from build123d import *

# Parameters (mm, degrees)
SKETCH1_W           = 5
SKETCH1_H           = 25
BOSS_EXTRUDE1_DEPTH = 258.5
SKETCH2_R           = 3
SKETCH2_R_2         = 1.5
CUT_EXTRUDE1_DEPTH  = 259.850342862


with BuildPart() as part:
    # Sketch1 → Boss-Extrude1 (new body)
    with BuildSketch(Plane.XY):
        Rectangle(SKETCH1_W, SKETCH1_H)
    extrude(amount=BOSS_EXTRUDE1_DEPTH)

    # Sketch2 → Cut-Extrude1 (cut, through all)
    with BuildSketch(Plane(origin=(2.5, 0, 0), x_dir=(0, 0, -1), z_dir=(1, 0, 0))):
        with Locations((-12.5, 0)):
            Circle(SKETCH2_R)
        with Locations((-246, 0)):
            Circle(SKETCH2_R_2)
        with Locations((-228, 0)):
            Circle(SKETCH2_R_2)
        with Locations((-48.5, 0)):
            Circle(SKETCH2_R_2)
        with Locations((-31.5, 0)):
            Circle(SKETCH2_R_2)
        with BuildLine():
            Line((-12.5, 12.5), (5.5, 12.5))
            Line((5.5, 12.5), (5.5, -12.5))
            Line((5.5, -12.5), (-12.5, -12.5))
            ThreePointArc((-12.5, -12.5), (0, 0), (-12.5, 12.5))
        make_face()
        Polygon((-257.716878365, 0), (-250.5, 12.5), (-258.5, 12.5), (-258.5, -12.5), (-250.5, -12.5), align=None)
    extrude(amount=-CUT_EXTRUDE1_DEPTH, mode=Mode.SUBTRACT)


solid = part.part
Design review of the part built by this model. Coordinates are the model's own, in mm. Coordinates: 2 decimals unless noted, no trailing zeros. Loops run counter-clockwise (first coordinate to the right, second up) from the corner with the lowest first, then second, coordinate; pieces in that order, holes last. Notation, with made-up numbers: (1.25, 88.5) - (11.25, 88.5) arc R12 ccw to (11.25, 95.5) - close; hole circle Ø2 at (63.5, 35). An arc over 180 degrees is marked (long way). Use CSV: the item, a comma, the result in double quotes. Start each with the question number.
1. Clearance check with flat-ended pins moving along their axes: pin 1 (1 mm diameter, centred on x = -0.5, y = -2.5, fed in from -Z); pin 2 (5.5 mm diameter, centred on y = 0, z = 12.5, fed in from +X); pin 3 (1 mm diameter, centred on x = 0, y = 8.5, fed in from +Z); pin 4 (1.5 mm diameter, centred on x = 2, y = -1.5, fed in from -Z). State where each tip first meets the part, or that it passes through.
2. Mouldability with a two-part tool opening along Y and no side actions: class faces 1 (the cylindrical face through (0, -1.8, 14.9)), 2 (the flat face through (0.035, -6.337, 254.058)), 3 (the flat face through (-2.5, 0, 127)) as released by +Y, released by -Y, zero draft, split by the parting line, or undercut.
3. Add section B-B on y = -8.75. Give the boundary of the cut face in (x, z).
4. Add section A-A on x = -1.4. Give the boundary of the cut face in (y, z), plus the area to 3 significant figures.
5. To check wall thickness, follow probe 1 along Y at (x, z) = (-1.3, 31.5); probe 2 along Z at (x, y) = (-1.6, -0.5); probe 3 along Z at (x, y) = (0.95, 1). State the ranges of each line that lie inside material, in increasing order.
Resolved:
1,pin 1,"z = 0.16"
1,pin 2,"through"
1,pin 3,"z = 253.1"
1,pin 4,"z = 0.02"
2,face 1,"undercut"
2,face 2,"released by -Y"
2,face 3,"zero draft"
3,outline,"(-2.5, 3.57) - (2.5, 3.57) - (2.5, 252.67) - (-2.5, 252.67) - close"
4,outline,"(-12.5, 12.5) arc R12.5 ccw to (12.5, 12.5) - (12.5, 250.5) - (0, 257.72) - (-12.5, 250.5) - close; hole circle Ø6 at (0, 12.5); hole circle Ø3 at (0, 31.5); hole circle Ø3 at (0, 48.5); hole circle Ø3 at (0, 228); hole circle Ø3 at (0, 246)"
4,area,"6,230 mm2"
5,probe 1,"-12.5 to -1.5, 1.5 to 12.5"
5,probe 2,"0.01 to 9.54, 15.46 to 30.09, 32.91 to 47.09, 49.91 to 226.59, 229.41 to 244.59, 247.41 to 257.43"
5,probe 3,"0.04 to 9.67, 15.33 to 30.38, 32.62 to 47.38, 49.62 to 226.88, 229.12 to 244.88, 247.12 to 257.14"
